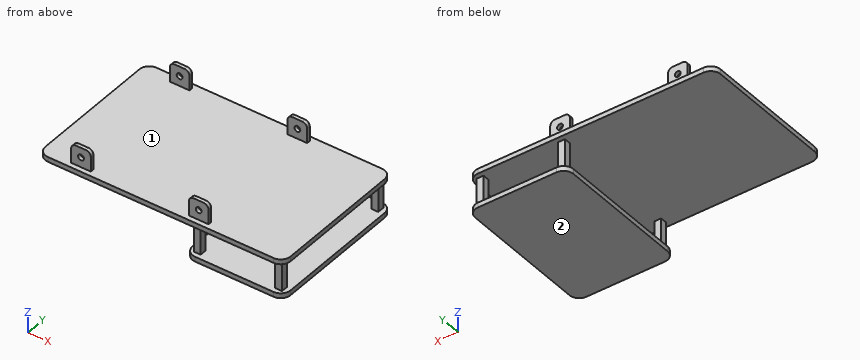
```python
from build123d import *

# Parameters (mm, degrees)
SKETCH1_W               = 250
SKETCH1_H               = 150
BOSS_EXTRUDE1_DEPTH     = 5
SKETCH1_3_W             = 20
SKETCH1_3_H             = 3.633461532
BOSS_EXTRUDE2_DEPTH     = 25
SKETCH2_R               = 3
CUT_EXTRUDE1_DEPTH      = 6
CUT_EXTRUDE1_DEPTH_BACK = 146
FILLET1_R               = 5
FILLET2_R               = 10
SKETCH3_W               = 7
SKETCH3_H               = 7
BOSS_EXTRUDE3_DEPTH     = 30
BOSS_EXTRUDE5_DEPTH     = 5
FILLET4_R               = 10


with BuildPart() as part:
    # Sketch1 → Boss-Extrude1 (new body)
    with BuildSketch(Plane.XY):
        with Locations((125, 75)):
            Rectangle(SKETCH1_W, SKETCH1_H)
    extrude(amount=BOSS_EXTRUDE1_DEPTH)

    # Sketch1<3> → Boss-Extrude2 (add)
    with BuildSketch(Plane.XY):
        with Locations((160, 6.816730766)):
            Rectangle(SKETCH1_3_W, SKETCH1_3_H)
        with Locations((40, 143.183269234)):
            Rectangle(SKETCH1_3_W, SKETCH1_3_H)
        with Locations((160, 143.183269234)):
            Rectangle(SKETCH1_3_W, SKETCH1_3_H)
        with Locations((40, 6.816730766)):
            Rectangle(SKETCH1_3_W, SKETCH1_3_H)
    extrude(amount=BOSS_EXTRUDE2_DEPTH)

    # Sketch2 → Cut-Extrude1 (cut, two sides)
    with BuildSketch(Plane.XZ.offset(-5)) as cut_extrude1_sk:
        with Locations((40, 15.1)):
            Circle(SKETCH2_R)
        with Locations((160, 15.1)):
            Circle(SKETCH2_R)
    extrude(amount=CUT_EXTRUDE1_DEPTH, mode=Mode.SUBTRACT)
    extrude(cut_extrude1_sk.sketch, amount=-CUT_EXTRUDE1_DEPTH_BACK, mode=Mode.SUBTRACT)

    # Fillet1
    fillet1_edges = [part.edges().sort_by_distance(p)[0] for p in [
        (50, 143.183269234, 25),
        (30, 143.183269234, 25),
        (30, 6.816730766, 25),
        (50, 6.816730766, 25),
        (150, 6.816730766, 25),
        (170, 6.816730766, 25),
        (170, 143.183269234, 25),
        (150, 143.183269234, 25),
    ]]
    fillet(fillet1_edges, radius=FILLET1_R)

    # Fillet2
    fillet2_edges = [part.edges().sort_by_distance(p)[0] for p in [
        (0, 0, 2.5),
        (0, 150, 2.5),
        (250, 150, 2.5),
        (250, 0, 2.5),
    ]]
    fillet(fillet2_edges, radius=FILLET2_R)

    # Sketch3 → Boss-Extrude3 (add)
    with BuildSketch(Plane(origin=(0, 0, 0), x_dir=(-1, 0, 0), z_dir=(0, 0, -1))):
        with Locations((-241.5, 141.5)):
            Rectangle(SKETCH3_W, SKETCH3_H)
        with Locations((-241.5, 8.5)):
            Rectangle(SKETCH3_W, SKETCH3_H)
        with Locations((-158.5, 8.5)):
            Rectangle(SKETCH3_W, SKETCH3_H)
        with Locations((-158.5, 141.5)):
            Rectangle(SKETCH3_W, SKETCH3_H)
    extrude(amount=BOSS_EXTRUDE3_DEPTH)

    # Sketch10 → Boss-Extrude5 (add)
    with BuildSketch(Plane(origin=(0, 0, -30), x_dir=(-1, 0, 0), z_dir=(0, 0, -1))):
        with BuildLine():
            Line((-150, 150), (-150, 0))
            Line((-150, 0), (-240, 0))
            ThreePointArc((-240, 0), (-247.071067812, 2.928932188), (-250, 10))
            Line((-250, 10), (-250, 140))
            ThreePointArc((-250, 140), (-247.071067812, 147.071067812), (-240, 150))
            Line((-240, 150), (-150, 150))
        make_face()
    extrude(amount=BOSS_EXTRUDE5_DEPTH)

    # Fillet4
    fillet4_edges = [part.edges().sort_by_distance(p)[0] for p in [
        (150, 150, -32.5),
        (150, 0, -32.5),
    ]]
    fillet(fillet4_edges, radius=FILLET4_R)


solid = part.part
```
Geometry check sheet. Reference: the model listing, model coordinates, mm. Face numbers are marked on the shaded views. Coordinates: 2 decimals unless noted, no trailing zeros. Write each loop counter-clockwise with the first axis right and the second up, starting at its lowest first coordinate (ties: lowest second). Pieces come first, ordered by that corner, then holes. Notation, with made-up numbers: M 8.25,62.5 L 64.25,62.5 A24 cw 64.25,96.5 Z; hole C -39.75,6 d3. An arc over 180 degrees is marked long. Use one line per item in the form item = value. Start each with the question number.
1) Go/stop test with flat-tipped pins: pin 1 Ø1.8 at (y, z) = (142.5, 13) entering from -X; pin 2 Ø12 at (x, y) = (140, 42.5) entering from -Z; pin 3 Ø16 at (x, z) = (38, 18.5) entering from -Y; pin 4 Ø10 at (y, z) = (16, -0.5) entering from +X. Record where each tip stops, or that it passes through.
2) Section check B-B on y = 129.5. Enter the section's corners in (x, z), and give its area (3 significant figures).
3) Section check D-D on z = 15.1. State how many separate pieces and enclosed holes the cut face has, and give its area (3 significant figures).
4) Section check C-C on z = -26.5. Enter the section's corners in (x, y), and give its area (3 significant figures).
5) Section check A-A on x = 40. Enter the section's corners in (y, z), and give its area (3 significant figures).
6) Thickness scan on probe 1 along Y at (x, z) = (48, 16.5); probe 2 along Z at (x, y) = (151.5, 90); probe 3 along X at (y, z) = (7, 15). Record the ranges inside material, lowest first. Write a range as from..to.
7) Release check for a two-part mould opening along Y. For the marked faces 1 and 2 record: pulls with the +Y half, pulls with the -Y half, needs draft (parallel to the pull), parting line crosses it, or undercut.
Responses:
q1.pin_1 = 30
q1.pin_2 = 0
q1.pin_3 = 5
q1.pin_4 = 250
q2.outline = M 0,0 L 250,0 L 250,5 L 0,5 Z; M 150,-35 L 250,-35 L 250,-30 L 150,-30 Z
q2.area = 1,750 mm2
q3.separate_pieces = 8
q3.enclosed_holes = 0
q3.area = 203 mm2
q4.outline = M 155,5 L 162,5 L 162,12 L 155,12 Z; M 155,138 L 162,138 L 162,145 L 155,145 Z; M 238,5 L 245,5 L 245,12 L 238,12 Z; M 238,138 L 245,138 L 245,145 L 238,145 Z
q4.area = 196 mm2
q5.outline = M 0,0 L 150,0 L 150,5 L 145,5 L 145,12.1 L 141.37,12.1 L 141.37,5 L 8.63,5 L 8.63,12.1 L 5,12.1 L 5,5 L 0,5 Z; M 5,18.1 L 8.63,18.1 L 8.63,25 L 5,25 Z; M 141.37,18.1 L 145,18.1 L 145,25 L 141.37,25 Z
q5.area = 852 mm2
q6.probe_1 = 5..8.63, 141.37..145
q6.probe_2 = -35..-30, 0..5
q6.probe_3 = 30..37, 43..50, 150..157, 163..170
q7.face_1 = undercut
q7.face_2 = needs draft
